Could you check a few things on this model? Use its own coordinates, in mm. A direction names the side the tool comes from. Round coordinates to 2 decimals unless told otherwise and drop trailing zeros. Write each loop counter-clockwise with the first axis right and the second up, starting at its lowest first coordinate (ties: lowest second). Pieces come first, ordered by that corner, then holes. Notation, with made-up numbers: (-39, 47) -> (-6, 47) arc R23 cw to (-6, 69) -> close; hole circle Ø6 at (16, 55). An arc over 180 degrees is marked (long way). Answer as CSV lines item,"result". Start each with the question number.
Q1. If we mould it in two halves opening along Z, with no side actions, what happens to faces 1 (the cylindrical face through (-26.235, 22.351, -0.34)), 2 (the cylindrical face through (-97, 0, 0)), 3 (the flat face through (-37, 31, 24.3)), 4 (the cylindrical face through (-74, 0, 0))? For each: pulls with the +Z half, pulls with the -Z half, needs draft (parallel to the pull), parting line crosses it, or undercut.
Q2. For faces 5 (the flat face through (-61.501, 38, 0)), 6 (the cylindrical face through (97, 0, 0)), 7 (the flat face through (-37, 31, -24.3)), which set-ups out of +Z, -Z, +X, -X, +Y, -Y let a thin tool reach every point of the face, with its end or its side?
Q3. Imagine slicing it at D-D on z = -18. Please give me the cut outline in (x, y).
Q4. If I drill on line 1 (Y direction, x = 0, z = -8); line 2 (X direction, y = 63, z = -6); line 3 (X direction, y = 95.5, z = 5), over which ranges is the centre line in solid material (lowest first)? Write a range as [from, to].
Q5. Imagine slicing it at B-B on x = 0. Please give me the cut outline in (y, z).
Q6. Imagine slicing it at A-A on z = 0. Please give me the cut outline in (x, y).
Q7. Imagine slicing it at C-C on y = 69. Please give me the cut outline in (x, z), and give its area (3 significant figures).
Q8. Will these pins go through, and if not, where does the flat tip stop? pin 1 Ø24.5 at (y, z) = (47, 8.5) entering from -X; pin 2 Ø14.5 at (y, z) = (40.5, -10) entering from +X; pin 3 Ø10 at (x, z) = (-23.5, 23.5) entering from +Y.
from build123d import *

# Parameters (mm, degrees)
SKETCH1_W           = 218.9988
SKETCH1_H           = 59.99988
BOSS_EXTRUDE1_DEPTH = 11.49985
CUT_EXTRUDE1_DEPTH  = 22.9997
SKETCH3_R           = 48.80102
BOSS_EXTRUDE2_DEPTH = 24.30018


with BuildPart() as part:
    # Sketch1 → Boss-Extrude1 (new, symmetric)
    with BuildSketch(Plane(origin=(0, 0, 0), x_dir=(1, 0, 0), z_dir=(0, 1, 0))):
        Rectangle(SKETCH1_W, SKETCH1_H)
    extrude(amount=BOSS_EXTRUDE1_DEPTH, both=True)

    # Sketch2 → Cut-Extrude1 (cut)
    with BuildSketch(Plane(origin=(0, 11.49985, 0), x_dir=(1, 0, 0), z_dir=(0, 1, 0))):
        with BuildLine():
            Line((-87.00135, 9.99998), (-84.00161, 9.99998))
            ThreePointArc((-84.00161, 9.99998), (-74.00163, 0), (-84.00161, -9.99998))
            Line((-84.00161, -9.99998), (-87.00135, -9.99998))
            ThreePointArc((-87.00135, -9.99998), (-97.00133, 0), (-87.00135, 9.99998))
        make_face()
        with BuildLine():
            Line((87.00135, 9.99998), (84.00161, 9.99998))
            ThreePointArc((84.00161, 9.99998), (74.00163, 0), (84.00161, -9.99998))
            Line((84.00161, -9.99998), (87.00135, -9.99998))
            ThreePointArc((87.00135, -9.99998), (97.00133, 0), (87.00135, 9.99998))
        make_face()
    extrude(amount=-CUT_EXTRUDE1_DEPTH, mode=Mode.SUBTRACT)

    # Sketch3 → Boss-Extrude2 (add, symmetric)
    with BuildSketch(Plane.XY):
        with BuildLine():
            Line((-61.50102, 63.5), (-61.50102, 11.49985))
            Line((-61.50102, 11.49985), (61.50102, 11.49985))
            Line((61.50102, 11.49985), (61.50102, 63.5))
            ThreePointArc((61.50102, 63.5), (0, 125.00102), (-61.50102, 63.5))
        make_face()
        with Locations(Location((0, 63.5, 0), (0, 0, 180))):
            Circle(SKETCH3_R, mode=Mode.SUBTRACT)
    extrude(amount=BOSS_EXTRUDE2_DEPTH, both=True)


solid = part.part
Checks:
1,face 1,"needs draft"
1,face 2,"undercut"
1,face 3,"pulls with the +Z half"
1,face 4,"undercut"
2,face 5,"+Z, -Z, -X, +Y"
2,face 6,"+Y, -Y"
2,face 7,"-Z, +X, -X, +Y"
3,outline,"(-109.5, -11.5) -> (109.5, -11.5) -> (109.5, 11.5) -> (61.5, 11.5) -> (61.5, 63.5) arc R61.5 ccw to (-61.5, 63.5) -> (-61.5, 11.5) -> (-109.5, 11.5) -> close; hole circle Ø97.6 at (0, 63.5)"
4,line 1,"[-11.5, 14.7], [112.3, 125]"
4,line 2,"[-61.5, -48.8], [48.8, 61.5]"
4,line 3,"[-52.52, -36.84], [36.84, 52.52]"
5,outline,"(-11.5, -30) -> (11.5, -30) -> (11.5, -24.3) -> (14.7, -24.3) -> (14.7, 24.3) -> (11.5, 24.3) -> (11.5, 30) -> (-11.5, 30) -> close; (112.3, -24.3) -> (125, -24.3) -> (125, 24.3) -> (112.3, 24.3) -> close"
6,outline,"(-109.5, -11.5) -> (-97, -11.5) -> (-97, 11.5) -> (-109.5, 11.5) -> close; (-74, -11.5) -> (74, -11.5) -> (74, 11.5) -> (61.5, 11.5) -> (61.5, 63.5) arc R61.5 ccw to (-61.5, 63.5) -> (-61.5, 11.5) -> (-74, 11.5) -> close; (97, -11.5) -> (109.5, -11.5) -> (109.5, 11.5) -> (97, 11.5) -> close; hole circle Ø97.6 at (0, 63.5)"
7,outline,"(-61.25, -24.3) -> (-48.49, -24.3) -> (-48.49, 24.3) -> (-61.25, 24.3) -> close; (48.49, -24.3) -> (61.25, -24.3) -> (61.25, 24.3) -> (48.49, 24.3) -> close"
7,area,"1,240 mm^2"
8,pin 1,"x = -61.5"
8,pin 2,"x = 61.5"
8,pin 3,"y = 122.15"
